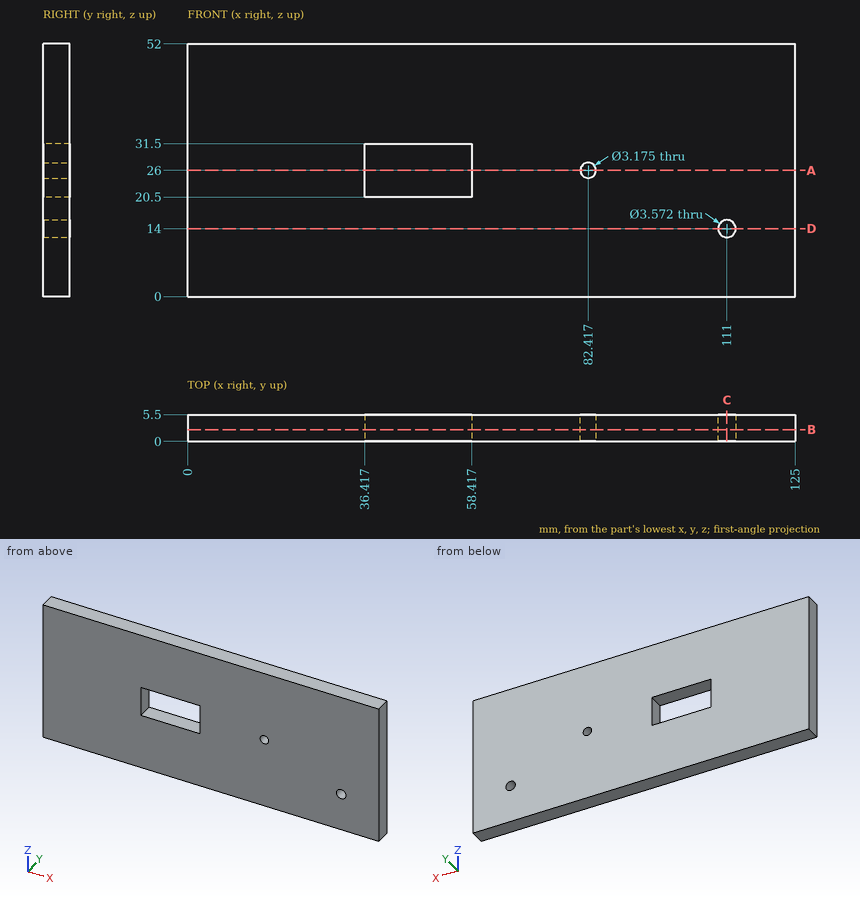
Part print with two shaded views. Sizes in mm from the minimum x, y, z corner. Coordinates: 2 decimals unless noted, no trailing zeros. Loops run counter-clockwise (first coordinate to the right, second up) from the corner with the lowest first, then second, coordinate; pieces in that order, holes last. Notation, with made-up numbers: (46, 6.25) - (97, 6.25) arc R17 ccw to (97, 37.25) - close; hole circle Ø10 at (6.25, -15). An arc over 180 degrees is marked (long way). Write each question's results on one line, items separated by ' | '. Start each with the question number.
Q1. Slice it at C-C on x = 111. Give the cut face in (y, z), and give its area (3 significant figures).
Q2. Slice it at D-D on z = 14. Give the cut face in (x, y).
Q3. Probe line 1 along Z through (x, y) = (111, 2.6); line 2 along X through (y, z) = (5.1, 24); line 3 along Z through (x, y) = (110, 2.1). List the from-to ranges inside material, lowest first.
Q4. Slice it at A-A on z = 26. Give the cut face in (x, y).
Q5. Slice it at B-B on y = 2.4. Give the cut face in (x, z) (1 decimal), and give its area (3 significant figures).
Answer:
1) outline: (0, 0) - (5.5, 0) - (5.5, 12.21) - (0, 12.21) - close; (0, 15.79) - (5.5, 15.79) - (5.5, 52) - (0, 52) - close | area: 266 mm2
2) outline: (0, 0) - (109.21, 0) - (109.21, 5.5) - (0, 5.5) - close; (112.79, 0) - (125, 0) - (125, 5.5) - (112.79, 5.5) - close
3) line 1: z = 0 to 12.21, 15.79 to 52 | line 2: x = 0 to 36.42, 58.42 to 125 | line 3: z = 0 to 12.52, 15.48 to 52
4) outline: (0, 0) - (36.42, 0) - (36.42, 5.5) - (0, 5.5) - close; (58.42, 0) - (80.83, 0) - (80.83, 5.5) - (58.42, 5.5) - close; (84, 0) - (125, 0) - (125, 5.5) - (84, 5.5) - close
5) outline: (0, 0) - (125, 0) - (125, 52) - (0, 52) - close; hole (36.4, 20.5) - (58.4, 20.5) - (58.4, 31.5) - (36.4, 31.5) - close; hole circle Ø3.2 at (82.4, 26); hole circle Ø3.6 at (111, 14) | area: 6,240 mm2
